Autodesk Inventor part; units mm, degrees
ref_plane "Work Plane1" through (-7, 48, -53) normal (0, 1, 0) x (1, 0, 0)
ref_plane "YZ Plane" through (0, 0, 0) normal (1, 0, 0) x (0, 1, 0)
ref_plane "XZ Plane" through (0, 0, 0) normal (0, 1, 0) x (-1, 0, 0)
sketch "Sketch2" plane through (0, 0, 0) normal (0, 1, 0) x (-1, 0, 0)
  line L0 (2, 0) -> (58, 0)
  line L1 (60, -2) -> (60, -58)
  line L2 (58, -60) -> (2, -60)
  line L3 (0, -58) -> (0, -2)
  line L4 (48, -46) -> (48, -14)
  line L5 (46, -12) -> (14, -12)
  line L6 (12, -14) -> (12, -46)
  line L7 (14, -48) -> (46, -48)
  arc A0 (60, -2) -> (58, 0) centre (58, -2) ccw
  arc A1 (58, -60) -> (60, -58) centre (58, -58) ccw
  arc A2 (0, -58) -> (2, -60) centre (2, -58) ccw
  arc A3 (2, 0) -> (0, -2) centre (2, -2) ccw
  arc A4 (14, -12) -> (12, -14) centre (14, -14) ccw
  arc A5 (12, -46) -> (14, -48) centre (14, -46) ccw
  arc A6 (46, -48) -> (48, -46) centre (46, -46) ccw
  arc A7 (48, -14) -> (46, -12) centre (46, -14) ccw
  point P0 (0, 0)
  point P1 (60, -60)
  point P2 (60, 0)
  point P3 (0, -60)
  dimension "d9" = 60
  dimension "d10" = 60
  dimension "d11" = 12
  dimension "d12" = 2
extrude "Extrusion2" add sketch "Sketch2" along normal blind 2
sketch "Sketch3" plane through (0, 2, 0) normal (0, 1, 0) x (1, 0, 0)
  circle A0 centre (-53, 7) radius 4
  circle A1 centre (-7, 7) radius 4
  circle A2 centre (-53, 53) radius 4
  circle A3 centre (-7, 53) radius 4
  line L0 (-58, 0) -> (-2, 0)
  line L1 (-60, 58) -> (-60, 2)
  line L2 (-2, 60) -> (-58, 60)
  line L3 (0, 2) -> (0, 58)
  point P0 (0, 0)
  dimension "d15" = 8
  dimension "d16" = 8
  dimension "d17" = 8
  dimension "d18" = 8
  dimension "d19" = 7
  dimension "d20" = 7
  dimension "d21" = 7
  dimension "d22" = 7
  dimension "d23" = 7
  dimension "d24" = 7
  dimension "d25" = 7
  dimension "d26" = 7
extrude "Extrusion4" add sketch "Sketch3" along normal blind 46
ref_plane "Work Plane1" through (-7, 48, -53) normal (0, 1, 0) x (1, 0, 0)
sketch "Sketch5" plane through (-7, 48, -53) normal (0, 1, 0) x (1, 0, 0)
  circle A0 centre (-46, 0) radius 4
  circle A1 centre (-46, 0) radius 1.25
  circle A2 centre (0, 0) radius 4
  circle A3 centre (0, 0) radius 1.25
  circle A4 centre (0, -46) radius 4
  circle A5 centre (0, -46) radius 1.25
  circle A6 centre (-46, -46) radius 4
  circle A7 centre (-46, -46) radius 1.25
  point P0 (7, -53)
  dimension "d36" = 2.5
  dimension "d37" = 2.5
  dimension "d38" = 2.5
  dimension "d39" = 2.5
extrude "Extrusion5" cut sketch "Sketch5" against normal blind 5 contours A1 | A3 | A5 | A7
properties part number "lidar base"
The model under review builds one solid part; all positions refer to its coordinate system, in mm. A direction names the side the tool comes from. Coordinates: 2 decimals unless noted, no trailing zeros. Write each loop counter-clockwise with the first axis right and the second up, starting at its lowest first coordinate (ties: lowest second). Pieces come first, ordered by that corner, then holes. Notation, with made-up numbers: (72, 29.25) -> (99, 29.25) arc R12 cw to (99, 46.25) -> close; hole circle Ø10 at (-33, -30). An arc over 180 degrees is marked (long way). One line per item, written item: value. Start each with the question number.
Q1. Add section B-B, the plane x = -41.5. Give the boundary of the cut face in (y, z), then the cut area to 3 significant figures.
Q2. Clearance check with flat-ended pins moving along their axes: P1, Ø0.8, axis at x = -7, z = -53, coming from the +Y side; P2, Ø6, axis at x = -48.5, z = -45.5, coming from the +Y side. State where each tip first meets the part, or that it passes through.
Q3. Add section C-C, the plane z = -36.5. Give the boundary of the cut face in (x, y).
Q4. The part is to be moulded in two halves that separate along X. For faces 4 (the face through (-47.43, 0.99, -47.4)), 5 (the face through (0, 1, -30)), 6 (the face through (-54, 48, -52)), say which applies: +X half, -X half, draft (parallel to the pull), parting line (faces both ways), or undercut.
Q5. For faces 1 (the face through (-0.57, 0.99, -0.6)), 2 (the face through (-30, 1, -48)), 3 (the face through (-30, 2, -50)), list the 3-axis set-ups (+Z, -Z, +X, -X, +Y, -Y) from which the entire face can be reached by the end or side of a thin tool; tool diameter is ignored.
Q6. Add section D-D, the plane x = -7. Give the boundary of the cut face in (y, z), then the cut area to 3 significant figures.
Q7. Add section A-A, the plane y = 44. Give the boundary of the cut face in (x, z), then the cut area to 3 significant figures.
Q8. To check wall thickness, follow probe 1 along Z at (x, y) = (-53, 45.4); probe 2 along X at (y, z) = (12, -53). State the ranges of each line that lie inside material, in increasing order.
Response:
1. outline: (0, -60) -> (2, -60) -> (2, -48) -> (0, -48) -> close; (0, -12) -> (2, -12) -> (2, 0) -> (0, 0) -> close
1. area: 48.0 mm²
2. P1: y = 43
2. P2: y = 2
3. outline: (-60, 0) -> (-48, 0) -> (-48, 2) -> (-60, 2) -> close; (-12, 0) -> (0, 0) -> (0, 2) -> (-12, 2) -> close
4. face 4: undercut
4. face 5: +X half
4. face 6: draft
5. face 1: +Z, +X, +Y, -Y
5. face 2: +Y, -Y
5. face 3: +Y
6. outline: (0, -60) -> (2, -60) -> (2, -57) -> (48, -57) -> (48, -54.25) -> (43, -54.25) -> (43, -51.75) -> (48, -51.75) -> (48, -49) -> (2, -49) -> (2, -11) -> (48, -11) -> (48, -8.25) -> (43, -8.25) -> (43, -5.75) -> (48, -5.75) -> (48, -3) -> (2, -3) -> (2, 0) -> (0, 0) -> close
6. area: 831 mm²
7. outline: circle Ø8 at (-53, -53); circle Ø8 at (-53, -7); circle Ø8 at (-7, -53); circle Ø8 at (-7, -7); hole circle Ø2.5 at (-53, -53); hole circle Ø2.5 at (-53, -7); hole circle Ø2.5 at (-7, -53); hole circle Ø2.5 at (-7, -7)
7. area: 181 mm²
8. probe 1: -57 to -54.25, -51.75 to -49, -11 to -8.25, -5.75 to -3
8. probe 2: -57 to -49, -11 to -3
